```python
from build123d import *

# Parameters (mm, degrees)
BOSS_EXTRUDE1_DEPTH = 3.499999985
CIRPATTERN1_COUNT   = 20
SKETCH2_W           = 10.342329408
SKETCH2_H           = 1.5875


with BuildPart() as part:
    # Sketch1 → Boss-Extrude1 (new, symmetric)
    with BuildSketch(Plane(origin=(0, 0, 0), x_dir=(1, 0, 0), z_dir=(0, 1, 0))):
        with BuildLine():
            ThreePointArc((0.872060607, 8.659786465), (0.562967303, 8.148255135), (0, 7.947579308))
            ThreePointArc((0, 7.947579308), (-1.243275317, -7.849731418), (2.45593707, 7.55859709))
            ThreePointArc((2.45593707, 7.55859709), (1.982535589, 7.923417607), (1.846642263, 8.505427895))
            ThreePointArc((1.846642263, 8.505427895), (1.749626992, 8.862101959), (1.434119122, 9.054671776))
            ThreePointArc((1.434119122, 9.054671776), (1.074545959, 8.969024291), (0.872060607, 8.659786465))
        make_face()
    boss_extrude1 = extrude(amount=BOSS_EXTRUDE1_DEPTH, both=True)

    # CirPattern1: Boss-Extrude1 ×20 about axis
    cirpattern1_axis = Axis((0, 0, 0), (0, 1, 0))
    for i in range(1, CIRPATTERN1_COUNT):
        add(boss_extrude1.rotate(cirpattern1_axis, i * 360 / CIRPATTERN1_COUNT))

    # Sketch2 → Revolve3 (revolve)
    with BuildSketch(Plane(origin=(0, 0, 0), x_dir=(0, 0, -1), z_dir=(1, 0, 0)), mode=Mode.PRIVATE) as revolve3_sk:
        with Locations((5.171164704, 4.293749985)):
            Rectangle(SKETCH2_W, SKETCH2_H)
    revolve3 = revolve(revolve3_sk.sketch.rotate(Axis((0, 3.3, 0), (0, -1, 0)), 180), axis=Axis((0, 3.3, 0), (0, -1, 0)))

    # Mirror1: Revolve3 across plane
    add(revolve3.mirror(Plane.ZX))

    # Sketch5 → Revolve4 (revolve)
    with BuildSketch(Plane.XY, mode=Mode.PRIVATE) as revolve4_sk:
        Polygon((0, -5.087499985), (13.500000032, -5.087499985), (13.500000032, -6.674999985), (12.5, -6.674999985), (12.5, -13.674999955), (0, -13.674999955), align=None)
    revolve(revolve4_sk.sketch.rotate(Axis((0, -13.674999955, 0), (0, 1, 0)), 90), axis=Axis((0, -13.674999955, 0), (0, 1, 0)))


solid = part.part
```
The model under review builds one solid part; all positions refer to its coordinate system, in mm. A direction names the side the tool comes from. Give positions to 0.01 mm unless a question says otherwise; leave off trailing zeros. Write each loop counter-clockwise with the first axis right and the second up, starting at its lowest first coordinate (ties: lowest second). Pieces come first, ordered by that corner, then holes. Notation, with made-up numbers: M -19.75,39 L 0.25,39 A18 cw 0.25,68 Z; hole C -11.75,-3 d4. An arc over 180 degrees is marked long. Answer in a Markdown table with one row per item.
Item 1: Add section A-A on x = 9.75. Give the boundary of the cut face in (y, z) (1 decimal), plus the area to 3 significant figures.
Check sheet entries:
| item | result |
|---|---|
| outline | M -13.7,-7.8 L -6.7,-7.8 L -6.7,-9.3 L -5.1,-9.3 L -5.1,-3.4 L -3.5,-3.4 L -3.5,3.4 L -5.1,3.4 L -5.1,9.3 L -6.7,9.3 L -6.7,7.8 L -13.7,7.8 Z; M 3.5,-3.4 L 5.1,-3.4 L 5.1,3.4 L 3.5,3.4 Z |
| area | 161 mm2 |
Item 2: Draft analysis for pull direction Y (two halves, no side actions). For faces 4 (the face through (9, -6.675, -9)), 5 (the face through (8, 3.5, -3)), 6 (the face through (0, 5.087, 0)), 7 (the face through (8, -3.5, -3)), state which applies: +Y half, -Y half, draft (parallel to the pull), parting line (faces both ways), or undercut.
Check sheet entries:
| item | result |
|---|---|
| face 4 | -Y half |
| face 5 | undercut |
| face 6 | +Y half |
| face 7 | undercut |
Item 3: For line 1 along Y through (x, z) = (-3, 9.25) (1 decimal); line 2 along Y through (x, z) = (-0.75, 10.75) (1 decimal); line 3 along Z through (x, y) = (4, 3), list the stretches that pass through material, from the lowest coordinate up.
Check sheet entries:
| item | result |
|---|---|
| line 1 | -13.7 to -3.5, 3.5 to 5.1 |
| line 2 | -13.7 to -5.1 |
| line 3 | -8.22 to 8.22 |
Item 4: Add section B-B on z = 10. Give the boundary of the cut face in (x, y) (1 decimal), plus the area to 3 significant figures.
Check sheet entries:
| item | result |
|---|---|
| outline | M -9.1,-6.7 L -7.5,-6.7 L -7.5,-13.7 L 7.5,-13.7 L 7.5,-6.7 L 9.1,-6.7 L 9.1,-5.1 L 2.6,-5.1 L 2.6,-3.5 L -2.6,-3.5 L -2.6,-5.1 L -9.1,-5.1 Z; M -2.6,3.5 L 2.6,3.5 L 2.6,5.1 L -2.6,5.1 Z |
| area | 151 mm2 |
Item 5: Tool access review of faces 1 (the face through (8, -5.087, 7)), 2 (the face through (-3.755, -10.224, -11.923)), 3 (the face through (8.215, -5.892, 10.713)): name each direction out of +Z, -Z, +X, -X, +Y, -Y from which nothing blocks a thin tool from reaching the whole face with its end or side.
Check sheet entries:
| item | result |
|---|---|
| face 1 | +Y |
| face 2 | -Y |
| face 3 | +Y, -Y |
Item 6: For P1, Ø6, axis at x = 3, y = -10.5, coming from the +Z side; P2, Ø8, axis at x = -5.5, y = -8.5, coming from the +Z side; P3, Ø3, axis at x = 7.5, y = -5, coming from the +Z side, all flat-tipped, find the tip position at first contact; note any pin that passes through.
Check sheet entries:
| item | result |
|---|---|
| P1 | z = 12.5 |
| P2 | z = 13.36 |
| P3 | z = 12.09 |
Item 7: Add section C-C on x = -11.25. Give the boundary of the cut face in (y, z) (1 decimal), plus the area to 4 significant figures.
Check sheet entries:
| item | result |
|---|---|
| outline | M -13.7,-5.4 L -6.7,-5.4 L -6.7,-7.5 L -5.1,-7.5 L -5.1,7.5 L -6.7,7.5 L -6.7,5.4 L -13.7,5.4 Z |
| area | 100.0 mm2 |
